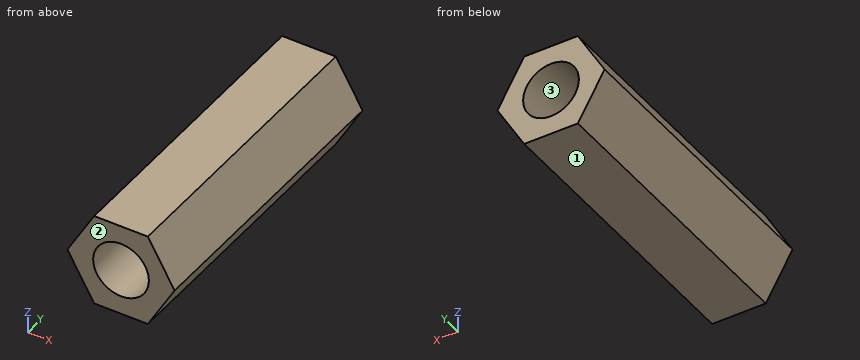
```python
from build123d import *

# Parameters (mm, degrees)
CROQUIS1_R              = 1.5
SALIENTE_EXTRUIR1_DEPTH = 6
SKETCH_1_R              = 1.5
EXTRUDE_1_DEPTH         = 4


with BuildPart() as part:
    # Croquis1 → Saliente-Extruir1 (new, symmetric)
    with BuildSketch(Plane(origin=(0, 0, 0), x_dir=(1, 0, 0), z_dir=(0, 1, 0))):
        Polygon((1.443375673, -2.5), (2.886751346, 0), (1.443375673, 2.5), (-1.443375673, 2.5), (-2.886751346, 0), (-1.443375673, -2.5), align=None)
        with Locations(Location((0, 0, 0), (0, 0, 270))):
            Circle(CROQUIS1_R, mode=Mode.SUBTRACT)
    extrude(amount=SALIENTE_EXTRUIR1_DEPTH, both=True)

    # 草图1 → 凸台-拉伸1 (add)
    with BuildSketch(Plane(origin=(0, 6, 0), x_dir=(1, 0, 0), z_dir=(0, 1, 0))):
        Polygon((-1.443375673, -2.5), (1.443375673, -2.5), (2.886751346, 0), (1.443375673, 2.5), (-1.443375673, 2.5), (-2.886751346, 0), align=None)
        with Locations(Location((0, 0, 0), (0, 0, 270))):
            Circle(SKETCH_1_R, mode=Mode.SUBTRACT)
    extrude(amount=EXTRUDE_1_DEPTH)


solid = part.part
```
Geometry check sheet. Reference: the model listing, model coordinates, mm. Face numbers are marked on the shaded views. Give positions to 0.01 mm unless a question says otherwise; leave off trailing zeros. Loops run counter-clockwise (first coordinate to the right, second up) from the corner with the lowest first, then second, coordinate; pieces in that order, holes last. Notation, with made-up numbers: M 29.5,52 L 36.5,52 A13 cw 36.5,77 Z; hole C 74,-27.75 d7. An arc over 180 degrees is marked long. Answer as CSV lines item,"result".
Item 1: Cross-section at D-D on x = 1.9. Record the cut outline in (y, z).
Values:
outline,"M -6,-1.71 L 10,-1.71 L 10,1.71 L -6,1.71 Z"
Item 2: Cross-section at C-C on y = 7.75. Record the cut outline in (x, z), and give its area (3 significant figures).
Values:
outline,"M -2.89,0 L -1.44,-2.5 L 1.44,-2.5 L 2.89,0 L 1.44,2.5 L -1.44,2.5 Z; hole C 0,0 d3"
area,"14.6 mm²"
Item 3: Material ranges on line 1 (X direction, y = 3.75, z = -0.4); line 2 (Z direction, x = 1.2, y = 9); line 3 (Z direction, x = 0.9, y = -3.75), recorded low to high.
Values:
line 1,"x = -2.66 to -1.45, 1.45 to 2.66"
line 2,"z = -2.5 to -0.9, 0.9 to 2.5"
line 3,"z = -2.5 to -1.2, 1.2 to 2.5"
Item 4: Cross-section at B-B on z = 0.6. Record the cut outline in (x, y), and give its area (3 significant figures).
Values:
outline,"M -2.54,-6 L -1.37,-6 L -1.37,10 L -2.54,10 Z; M 1.37,-6 L 2.54,-6 L 2.54,10 L 1.37,10 Z"
area,"37.3 mm²"
Item 5: Cross-section at A-A on x = 0. Record the cut outline in (y, z).
Values:
outline,"M -6,-2.5 L 10,-2.5 L 10,-1.5 L -6,-1.5 Z; M -6,1.5 L 10,1.5 L 10,2.5 L -6,2.5 Z"
Item 6: Release check for a two-part mould opening along Z. For the marked faces 1, 2 and 3 record: pulls with the +Z half, pulls with the -Z half, needs draft (parallel to the pull), parting line crosses it, or undercut.
Values:
face 1,"pulls with the -Z half"
face 2,"needs draft"
face 3,"undercut"
Item 7: Depth check by flat-ended pin: P1, Ø1.5, axis at y = -1, z = 1, coming from the +X side; P2, Ø2.5, axis at x = 0, z = 0, coming from the +Y side. Enter the tip coordinate at first touch or a pass-through.
Values:
P1,"stops at x = 2.74"
P2,"passes through"
